The listing builds one solid part. Answer for the finished solid, in the listing's coordinates (mm). Face numbers are marked on the shaded views. Round coordinates to 2 decimals unless told otherwise and drop trailing zeros. Write each loop counter-clockwise with the first axis right and the second up, starting at its lowest first coordinate (ties: lowest second). Pieces come first, ordered by that corner, then holes.
from build123d import *

# Parameters (mm, degrees)
SKETCH013_R     = 4.5
SKETCH013_R_2   = 1.75
SKETCH013_W     = 7
SKETCH013_H     = 7
PAD004_DEPTH    = 3
PAD_DEPTH       = 10
SKETCH015_R     = 1.75
POCKET005_DEPTH = 5
SKETCH004_R     = 1.75
POCKET006_DEPTH = 5
SKETCH014_R     = 1.75
POCKET007_DEPTH = 5
POCKET_DEPTH    = 2


with BuildPart() as part:
    # Sketch013 → Pad004 (new body)
    with BuildSketch(Plane.XY):
        Polygon((0, 65), (150, 64.999907), (150, -65), (0, -65), align=None)
        with Locations((20, 18)):
            Circle(SKETCH013_R, mode=Mode.SUBTRACT)
        with Locations((59, 18)):
            Circle(SKETCH013_R, mode=Mode.SUBTRACT)
        with Locations((20, -30)):
            Circle(SKETCH013_R, mode=Mode.SUBTRACT)
        with Locations((59, -30)):
            Circle(SKETCH013_R, mode=Mode.SUBTRACT)
        with Locations((146, 60.999907)):
            Circle(SKETCH013_R_2, mode=Mode.SUBTRACT)
        with Locations((146, -61)):
            Circle(SKETCH013_R_2, mode=Mode.SUBTRACT)
        with Locations((82.370022, 45.189481)):
            Circle(SKETCH013_R_2, mode=Mode.SUBTRACT)
        with Locations((134.63, 45.189481)):
            Circle(SKETCH013_R_2, mode=Mode.SUBTRACT)
        with Locations((82.271087, -46.110465)):
            Circle(SKETCH013_R_2, mode=Mode.SUBTRACT)
        with Locations((134.531066, -46.110465)):
            Circle(SKETCH013_R_2, mode=Mode.SUBTRACT)
        with Locations((90.500022, 44.539481)):
            Rectangle(SKETCH013_W, SKETCH013_H, mode=Mode.SUBTRACT)
        with Locations((108.500011, 44.519694)):
            Rectangle(SKETCH013_W, SKETCH013_H, mode=Mode.SUBTRACT)
        with Locations((126.5, 44.499907)):
            Rectangle(SKETCH013_W, SKETCH013_H, mode=Mode.SUBTRACT)
        with Locations((90.480235, 26.539492)):
            Rectangle(SKETCH013_W, SKETCH013_H, mode=Mode.SUBTRACT)
        with Locations((108.480224, 26.519705)):
            Rectangle(SKETCH013_W, SKETCH013_H, mode=Mode.SUBTRACT)
        with Locations((126.480213, 26.499918)):
            Rectangle(SKETCH013_W, SKETCH013_H, mode=Mode.SUBTRACT)
        with Locations((90.460448, 8.539503)):
            Rectangle(SKETCH013_W, SKETCH013_H, mode=Mode.SUBTRACT)
        with Locations((108.460437, 8.519716)):
            Rectangle(SKETCH013_W, SKETCH013_H, mode=Mode.SUBTRACT)
        with Locations((126.460426, 8.499929)):
            Rectangle(SKETCH013_W, SKETCH013_H, mode=Mode.SUBTRACT)
        with Locations((90.440661, -9.460486)):
            Rectangle(SKETCH013_W, SKETCH013_H, mode=Mode.SUBTRACT)
        with Locations((108.44065, -9.480273)):
            Rectangle(SKETCH013_W, SKETCH013_H, mode=Mode.SUBTRACT)
        with Locations((126.440639, -9.50006)):
            Rectangle(SKETCH013_W, SKETCH013_H, mode=Mode.SUBTRACT)
        with Locations((90.420874, -27.460475)):
            Rectangle(SKETCH013_W, SKETCH013_H, mode=Mode.SUBTRACT)
        with Locations((108.420863, -27.480262)):
            Rectangle(SKETCH013_W, SKETCH013_H, mode=Mode.SUBTRACT)
        with Locations((126.420852, -27.500049)):
            Rectangle(SKETCH013_W, SKETCH013_H, mode=Mode.SUBTRACT)
        with Locations((90.401087, -45.460465)):
            Rectangle(SKETCH013_W, SKETCH013_H, mode=Mode.SUBTRACT)
        with Locations((108.401076, -45.480251)):
            Rectangle(SKETCH013_W, SKETCH013_H, mode=Mode.SUBTRACT)
        with Locations((126.401066, -45.500038)):
            Rectangle(SKETCH013_W, SKETCH013_H, mode=Mode.SUBTRACT)
    extrude(amount=PAD004_DEPTH)

    # Sketch001 (on DatumPlane) → Pad (join)
    with BuildSketch(Plane.XY.offset(3)):
        Polygon((0, 55), (3, 55), (128, 55), (128, 52), (3, 52), (3, -62), (128, -62), (128, -65), (3, -65), (0, -65), align=None)
    extrude(amount=PAD_DEPTH)

    # Sketch015 → Pocket005 (cut)
    with BuildSketch(Plane.XZ.offset(65)):
        with Locations((25, 9.5)):
            Circle(SKETCH015_R)
        with Locations((75, 9.5)):
            Circle(SKETCH015_R)
        with Locations((125, 9.5)):
            Circle(SKETCH015_R)
    extrude(amount=-POCKET005_DEPTH, mode=Mode.SUBTRACT)

    # Sketch004 (on DatumPlane) → Pocket006 (cut, symmetric)
    with BuildSketch(Plane.XZ.offset(-55)):
        with Locations((25, 9.5)):
            Circle(SKETCH004_R)
        with Locations((75, 9.5)):
            Circle(SKETCH004_R)
        with Locations((125, 9.5)):
            Circle(SKETCH004_R)
    extrude(amount=POCKET006_DEPTH, both=True, mode=Mode.SUBTRACT)

    # Sketch014 → Pocket007 (cut)
    with BuildSketch(Plane.YZ):
        with Locations((45, 9.5)):
            Circle(SKETCH014_R)
        with Locations((-5, 9.5)):
            Circle(SKETCH014_R)
        with Locations((-55, 9.5)):
            Circle(SKETCH014_R)
    extrude(amount=POCKET007_DEPTH, mode=Mode.SUBTRACT)

    # Sketch → Pocket (cut)
    with BuildSketch(Plane.XY.offset(3.5)):
        Polygon((85.120022, 49.539508), (85.120022, 42.439481), (78.000011, 42.439481), (78.000011, -43.360465), (85.021087, -43.360465), (85.021087, -50.460443), (131.781066, -50.460443), (131.781066, -43.360465), (139.000011, -43.360465), (139.000011, 42.439481), (131.88, 42.439481), (131.88, 49.539508), align=None)
    extrude(amount=-POCKET_DEPTH, mode=Mode.SUBTRACT)


solid = part.part
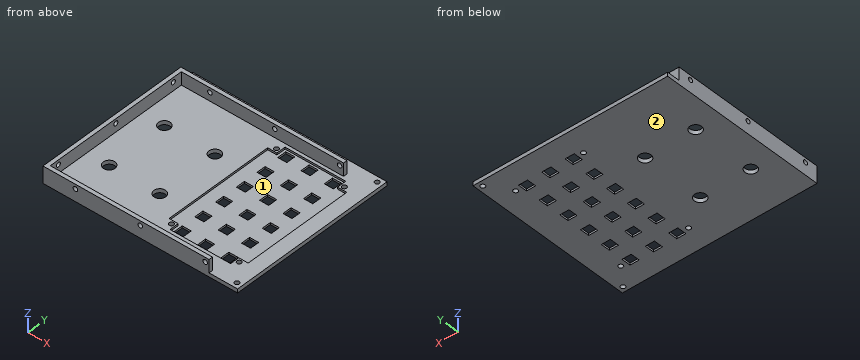
1. Section D-D on z = 5.5 is taken. Determine the outline of the cut face in (x, y).
Geometry says:
outline: (0, -65) - (128, -65) - (128, -62) - (3, -62) - (3, 52) - (128, 52) - (128, 55) - (0, 55) - close
2. Section A-A on y = 18 is taken. Determine the outline of the cut face in (x, z), plus the area to 4 significant figures.
Geometry says:
outline: (0, 0) - (15.5, 0) - (15.5, 3) - (3, 3) - (3, 13) - (0, 13) - close; (24.5, 0) - (54.5, 0) - (54.5, 3) - (24.5, 3) - close; (63.5, 0) - (150, 0) - (150, 3) - (139, 3) - (139, 1.5) - (78, 1.5) - (78, 3) - (63.5, 3) - close
area: 334.5 mm2
3. Given pin 1 (2 mm diameter, centred on y = -5, z = 9.5, fed in from -X); pin 2 (3 mm diameter, centred on x = 129, z = 5, fed in from -Y); pin 3 (3 mm diameter, centred on x = 30.5, y = 42.5, fed in from +Z), each flat-ended and moving along its own axis, determine where each tip first touches the part or whether it passes through.
Geometry says:
pin 1: passes through
pin 2: stops at y = -65
pin 3: stops at z = 3
4. For a pull along X with two mould halves and no side action, classify the marked faces 1 and 2 as released by +X, released by -X, zero draft, split by the parting line, or undercut.
Geometry says:
face 1: undercut
face 2: zero draft
5. Section C-C on y = -55 is taken. Determine the outline of the cut face in (x, z), plus the area to 4 significant figures.
Geometry says:
outline: (0, 0) - (150, 0) - (150, 3) - (3, 3) - (3, 7.75) - (0, 7.75) - close; (0, 11.25) - (3, 11.25) - (3, 13) - (0, 13) - close
area: 469.5 mm2
6. Section B-B on x = 20 is taken. Determine the outline of the cut face in (y, z).
Geometry says:
outline: (-65, 0) - (-34.5, 0) - (-34.5, 3) - (-62, 3) - (-62, 13) - (-65, 13) - close; (-25.5, 0) - (13.5, 0) - (13.5, 3) - (-25.5, 3) - close; (22.5, 0) - (65, 0) - (65, 3) - (55, 3) - (55, 13) - (52, 13) - (52, 3) - (22.5, 3) - close
7. Straight lines are drawn through the part: line 1 along Y through (x, z) = (134.63, 1.85); line 2 along Y through (x, z) = (20, 0.9); line 3 along Y through (x, z) = (115.5, 11.5). For each, find the intervals that lie inside material, in ascending order.
Geometry says:
line 1: y = -65 to -47.86, -44.36 to -43.36, 42.44 to 43.44, 46.94 to 65
line 2: y = -65 to -34.5, -25.5 to 13.5, 22.5 to 65
line 3: y = -65 to -62, 52 to 55
